Part model, mm, in its own coordinate system. A direction names the side the tool comes from. Round coordinates to 2 decimals unless told otherwise and drop trailing zeros. Write each loop counter-clockwise with the first axis right and the second up, starting at its lowest first coordinate (ties: lowest second). Pieces come first, ordered by that corner, then holes. Notation, with made-up numbers: M 21,0 L 57,0 A12 ccw 57,18 Z; hole C 3.25,38.25 d10. An arc over 180 degrees is marked long. Answer as a JSON object with one key per item and string values. Group by question number.
1. Band-saw the part on C-C, the plane z = 2.75. Count the separate pieces of the cut face and the enclosed holes in it, plus the area to 3 significant figures.
2. Drill centre lines: line 1 (Y direction, x = -41, z = 8.75); line 2 (X direction, y = 104.5, z = 14); line 3 (Y direction, x = -5, z = 6.5). Where is each one in solid material? Low to high. Write a range as from..to.
3. Band-saw the part on B-B, the plane y = 142. Write the cut outline in (x, z), plus the area to 3 significant figures.
4. Drop flat-ended pins along their axis: pin 1 (1 mm diameter, centred on x = 114, z = 9.5, fed in from -Y); pin 2 (8 mm diameter, centred on y = 164.5, z = 12.5, fed in from +X); pin 3 (3 mm diameter, centred on y = 77.5, z = 10.5, fed in from +X). Give the stop position or say it passes through.
5. Band-saw the part on A-A, the plane x = 0. Write the cut outline in (y, z), plus the area to 3 significant figures.
6. Two-plate mould, pull along Y, no slides. Class faces 4 (the face through (-47.908, 215.745, 7.395)), 5 (the face through (-36.825, -198.146, 5.67)), 6 (the face through (-50, -163, 0)): +Y half, -Y half, draft (parallel to the pull), parting line (faces both ways), or undercut.
7. Which spindle directions (+Z, -Z, +X, -X, +Y, -Y) get a long thin tool onto all of the face, cutting with end or side? Do faces 1 (the face through (-38.91, -175.23, 13.27)), 2 (the face through (3.68, -168.96, 7.4)), 3 (the face through (132, -106, 15)). Say none if no direction does.
Autodesk Inventor part; units mm, degrees
ref_plane "YZ Plane" through (0, 0, 0) normal (1, 0, 0) x (0, 1, 0)
ref_plane "XZ Plane" through (0, 0, 0) normal (0, 1, 0) x (-1, 0, 0)
ref_plane "XY Plane" through (0, 0, 0) normal (0, 0, 1) x (1, 0, 0)
sketch "Sketch1" plane through (0, 0, 0) normal (0, 0, 1) x (1, 0, 0)
  circle A0 centre (0, 0) radius 169
  circle A1 centre (0, 0) radius 221
  circle A2 centre (0, 0) radius 195 construction
  line L0 (0, 169) -> (0, 221) construction
  point P0 (0, 195)
  dimension "d17" = 390
  dimension "d18" = 52
extrude "Extrusion1" add sketch "Sketch1" along normal blind 15
sketch "Sketch2" plane through (0, 0, 15) normal (0, 0, 1) x (1, 0, 0)
  circle A0 centre (0, 0) radius 221 construction
  circle A1 centre (0, 0) radius 169 construction
  line L0 (0, 210.5) -> (0, 179.5) construction
  line L1 (0, 169) -> (0, 0) construction
  circle A2 centre (0, 0) radius 179.5
  circle A3 centre (0, 0) radius 210.5
  circle A4 centre (0, 0) radius 195 construction
  point P0 (0, 195)
  dimension "d19" = 390
  dimension "d4" = 31
extrude "Extrusion2" cut sketch "Sketch2" against normal blind 3.5
sketch "Sketch3" plane through (0, 0, 0) normal (0, 0, 1) x (1, 0, 0)
  circle A0 centre (0, 0) radius 169 construction
  circle A1 centre (0, 0) radius 221 construction
  circle A2 centre (0, 0) radius 179.5
  circle A3 centre (0, 0) radius 210.5
  circle A4 centre (0, 0) radius 221
  line L0 (0, 0) -> (0, -221) construction
  line L1 (0, 0) -> (43.115, -216.7535) construction
  line L2 (35.0187, -176.051) -> (41.0665, -206.4553) construction
  circle A5 centre (38.0426, -191.2531) radius 7
  dimension "d20" = 11.25
  dimension "d21" = 14
extrude "Extrusion3" cut sketch "Sketch3" along normal through all contours A5
pattern_circular "Circular Pattern2" count 8 over 157.5 about axis through (0, 0, 0) along (0, 0, -1) of "Extrusion3" both ways yes
sketch "Sketch5" plane through (0, 0, 0) normal (0, 0, -1) x (-1, 0, 0)
  circle A0 centre (0, 0) radius 169
  circle A1 centre (0, 0) radius 221
  line L0 (0, 0) -> (169, 0) construction
  arc A2 (168.9815, -2.4999) -> (168.9815, 2.4999) centre (169, 0) ccw
  dimension "d36" = 5
extrude "Extrusion4" cut sketch "Sketch5" against normal through all contours A0 A2
mirror "Mirror1" about plane through (0, 0, 0) normal (1, 0, 0) of "Extrusion4"
equation "\"d17\" = Шпил_пласт_НОС_диам_центров"
equation "\"d19\" = Шпил_пласт_НОС_диам_центров"
equation "\"BendReliefDepth\" = 0.5 * Thickness"
properties part number "ДМФ 021 кольцо прижимное нос v2.0"
Worked answers:
{
 "1": {"separate pieces": "1", "enclosed holes": "9", "area": "62,500 mm^2"},
 "2": {"line 1": "y = -217.16..-197.6, -184.91..-163.95, 163.95..217.16", "line 2": "x = -194.73..-182.73, -145.95..-132.82, 132.82..145.95, 182.73..194.73", "line 3": "y = -220.94..-168.93, 168.93..220.94"},
 "3": {"outline": "M -169.34,0 L -91.64,0 L -91.64,15 L -109.8,15 L -109.8,11.5 L -155.39,11.5 L -155.39,15 L -169.34,15 Z; M 91.64,0 L 169.34,0 L 169.34,15 L 155.39,15 L 155.39,11.5 L 109.8,11.5 L 109.8,15 L 91.64,15 Z", "area": "2,010 mm^2"},
 "4": {"pin 1": "stops at y = -189.63", "pin 2": "stops at x = 151.92", "pin 3": "stops at x = 207.52"},
 "5": {"outline": "M -221,0 L -169,0 L -169,15 L -179.5,15 L -179.5,11.5 L -210.5,11.5 L -210.5,15 L -221,15 Z; M 169,0 L 221,0 L 221,15 L 210.5,15 L 210.5,11.5 L 179.5,11.5 L 179.5,15 L 169,15 Z", "area": "1,340 mm^2"},
 "6": {"face 4": "parting line", "face 5": "undercut", "face 6": "draft"},
 "7": {"face 1": "+Z", "face 2": "+Z, -Z", "face 3": "+Z, +X, -X, +Y, -Y"}
}
